Verification items for the finished model (mm, model axes). Face numbers are marked on the shaded views. A direction names the side the tool comes from. Coordinates: 2 decimals unless noted, no trailing zeros. Order: outer loops, then holes, each group sorted by start corner. A loop starts at its lowest first (then second) coordinate and runs counter-clockwise, first axis right, second up.
Q1. Cross-section at B-B, the plane x = 3.5. Record the boundary of the cut face in (y, z), and give its area (3 significant figures).
Q2. Cross-section at D-D, the plane y = 5. Record the boundary of the cut face in (x, z), and give its area (3 significant figures).
Q3. Thickness scan on line 1 (Y direction, x = 28, z = -8.5); line 2 (X direction, y = 4.6, z = -3.5); line 3 (X direction, y = 5.35, z = -2.5). Record the ranges inside material, lowest first.
Q4. Cross-section at C-C, the plane z = -8.5. Record the boundary of the cut face in (x, y).
Q5. Set-up check for the marked faces 5 and 6: record each of +Z, -Z, +X, -X, +Y, -Y from which the full face is reachable in a straight line by a thin tool's end or side.
Q6. Cross-section at A-A, the plane y = 3. Record the boundary of the cut face in (x, z).
Q7. Draft check along Z on the marked faces 1, 2, 3 and 4. Enter one of: pulls with the +Z half, pulls with the -Z half, needs draft (parallel to the pull), parting line crosses it, or undercut.
Q8. Depth check by flat-ended pin: P1, Ø2, axis at x = 32, y = 0.5, coming from the -Z side. Enter the tip coordinate at first touch or a pass-through.
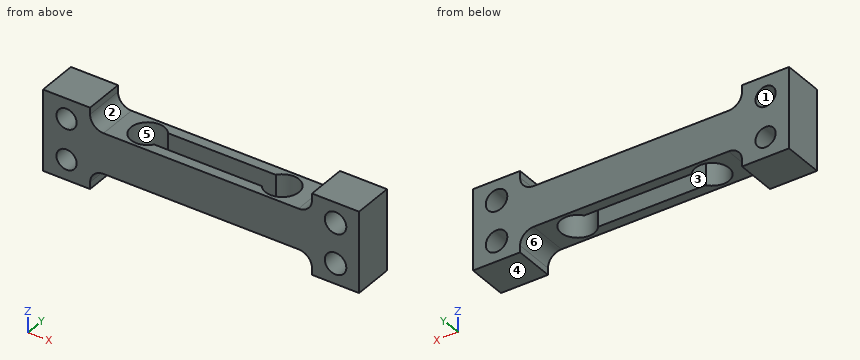
from build123d import *

# Parameters (mm, degrees)
SKETCH1_R           = 1.5
SKETCH1_R_2         = 1.6
BOSS_EXTRUDE2_DEPTH = 6
CUT_EXTRUDE1_DEPTH  = 49.228622207


with BuildPart() as part:
    # Sketch1 → Boss-Extrude2 (new body)
    with BuildSketch(Plane(origin=(0, 0, 0), x_dir=(1, 0, 0), z_dir=(0, 1, 0))):
        with BuildLine():
            Line((40, 0), (47, 0))
            Line((47, 0), (47, 12))
            Line((47, 12), (40, 12))
            Line((40, 12), (40, 11))
            ThreePointArc((40, 11), (39.414213562, 9.585786438), (38, 9))
            Line((38, 9), (9, 9))
            ThreePointArc((9, 9), (7.585786438, 9.585786438), (7, 11))
            Line((7, 11), (7, 12))
            Line((7, 12), (0, 12))
            Line((0, 12), (0, 0))
            Line((0, 0), (7, 0))
            Line((7, 0), (7, 1))
            ThreePointArc((7, 1), (7.585786438, 2.414213562), (9, 3))
            Line((9, 3), (38, 3))
            ThreePointArc((38, 3), (39.414213562, 2.414213562), (40, 1))
            Line((40, 1), (40, 0))
        make_face()
        with Locations(Location((3.5, 9, 0), (0, 0, 270))):
            Circle(SKETCH1_R, mode=Mode.SUBTRACT)
        with Locations(Location((3.5, 3, 0), (0, 0, 270))):
            Circle(SKETCH1_R, mode=Mode.SUBTRACT)
        with Locations(Location((43.5, 9, 0), (0, 0, 270))):
            Circle(SKETCH1_R_2, mode=Mode.SUBTRACT)
        with Locations(Location((43.5, 3, 0), (0, 0, 270))):
            Circle(SKETCH1_R_2, mode=Mode.SUBTRACT)
    extrude(amount=BOSS_EXTRUDE2_DEPTH)

    # Sketch2 → Cut-Extrude1 (cut, through all)
    with BuildSketch(Plane(origin=(0, 0, -9), x_dir=(-1, 0, 0), z_dir=(0, 0, -1))):
        with BuildLine():
            Line((-31.5, 4.5), (-15.5, 4.5))
            ThreePointArc((-15.5, 4.5), (-11, 3), (-15.5, 1.5))
            Line((-15.5, 1.5), (-31.5, 1.5))
            ThreePointArc((-31.5, 1.5), (-36, 3), (-31.5, 4.5))
        make_face()
    extrude(amount=-CUT_EXTRUDE1_DEPTH, mode=Mode.SUBTRACT)


solid = part.part
Check values:
1. outline: (0, -12) - (6, -12) - (6, -10.5) - (0, -10.5) - close; (0, -7.5) - (6, -7.5) - (6, -4.5) - (0, -4.5) - close; (0, -1.5) - (6, -1.5) - (6, 0) - (0, 0) - close
1. area: 36.0 mm2
2. outline: (0, -12) - (7, -12) - (7, -11) arc R2 cw to (9, -9) - (12, -9) - (12, -3) - (9, -3) arc R2 cw to (7, -1) - (7, 0) - (0, 0) - close; (15, -9) - (32, -9) - (32, -3) - (15, -3) - close; (35, -9) - (38, -9) arc R2 cw to (40, -11) - (40, -12) - (47, -12) - (47, 0) - (40, 0) - (40, -1) arc R2 cw to (38, -3) - (35, -3) - close; hole circle Ø3 at (3.5, -9); hole circle Ø3 at (3.5, -3); hole circle Ø3.2 at (43.5, -9); hole circle Ø3.2 at (43.5, -3)
2. area: 303 mm2
3. line 1: y = 0 to 1.5, 4.5 to 6
3. line 2: x = 0 to 2.09, 4.91 to 11.58, 15.42 to 31.58, 35.42 to 41.98, 45.02 to 47
3. line 3: x = 0 to 2.09, 4.91 to 7.68, 39.32 to 41.98, 45.02 to 47
4. outline: (0, 0) - (2.09, 0) - (2.09, 6) - (0, 6) - close; (4.91, 0) - (41.98, 0) - (41.98, 6) - (4.91, 6) - close; (45.02, 0) - (47, 0) - (47, 6) - (45.02, 6) - close; hole (15.5, 1.5) - (31.5, 1.5) arc R2.5 ccw (long way) to (31.5, 4.5) - (15.5, 4.5) arc R2.5 ccw (long way) to start
5. face 5: +Z, -Z
5. face 6: -Z, +Y, -Y
6. outline: (0, -12) - (7, -12) - (7, -11) arc R2 cw to (9, -9) - (11, -9) - (11, -3) - (9, -3) arc R2 cw to (7, -1) - (7, 0) - (0, 0) - close; (36, -9) - (38, -9) arc R2 cw to (40, -11) - (40, -12) - (47, -12) - (47, 0) - (40, 0) - (40, -1) arc R2 cw to (38, -3) - (36, -3) - close; hole circle Ø3 at (3.5, -9); hole circle Ø3 at (3.5, -3); hole circle Ø3.2 at (43.5, -9); hole circle Ø3.2 at (43.5, -3)
7. face 1: undercut
7. face 2: pulls with the +Z half
7. face 3: needs draft
7. face 4: pulls with the -Z half
8. P1: stops at z = -9
